from build123d import *

# Parameters (mm, degrees)
F1_DEPTH  = 26.8
F2_W      = 9.5
F2_H      = 26.8
F3_DEPTH  = 32.4
F4_W      = 53.02
F4_H      = 26.4
F5_DEPTH  = 15
F6_W      = 41.02
F6_H      = 26.4
F7_DEPTH  = 7
F8_W      = 33.1776287834
F8_H      = 14.4
F9_DEPTH  = 7
F10_W     = 16.1501816639
F10_H     = 14.4
F11_DEPTH = 7
F12_R     = 0.6930745825
F13_DEPTH = 5
F14_R     = 0.7453155857
F15_DEPTH = 5
F16_R     = 0.7584591481
F17_DEPTH = 5
F18_R     = 0.7431215043
F19_DEPTH = 5
F20_W     = 4
F20_H     = 9
F21_DEPTH = 5
F22_W     = 10
F22_H     = 13
F23_DEPTH = 1.5
F24_R     = 0.5
F25_R     = 2
F26_R     = 1
F27_DEPTH = 5
F28_R     = 1
F29_DEPTH = 5
F30_R     = 1
F31_DEPTH = 5
F32_R     = 1
F33_DEPTH = 5


with BuildPart() as f1:
    # F0 (on Front) → F1 (new body)
    with BuildSketch(Plane.XZ):
        Polygon((13.4, 0), (-13.4, 0), (-9.5, -6.25), (9.5, -6.25), align=None)
    extrude(amount=F1_DEPTH)

    # F2 (on face) → F3 (join)
    with BuildSketch(Plane(origin=(0, 0, -6.25), x_dir=(1, 0, 0), z_dir=(0, 0, -1))):
        Polygon((24, 42.91), (0, 42.91), (0, 26.8), (9.5, 26.8), (9.5, 0), (0, 0), (0, -16.11), (24, -16.11), align=None)
        with Locations((4.75, 13.4)):
            Rectangle(F2_W, F2_H)
    extrude(amount=F3_DEPTH)

    # F4 (on face) → F5 (cut)
    with BuildSketch(Plane.YZ.offset(24)):
        with Locations((-13.4, -22.45)):
            Rectangle(F4_W, F4_H)
    extrude(amount=-F5_DEPTH, mode=Mode.SUBTRACT)

    # F6 (on face) → F7 (cut)
    with BuildSketch(Plane.YZ.offset(9)):
        with Locations((-13.4, -22.45)):
            Rectangle(F6_W, F6_H)
    extrude(amount=-F7_DEPTH, mode=Mode.SUBTRACT)

    # F8 (on face) → F9 (cut)
    with BuildSketch(Plane.YZ.offset(9)):
        with Locations((-23.3211856083, -22.45)):
            Rectangle(F8_W, F8_H)
    extrude(amount=-F9_DEPTH, mode=Mode.SUBTRACT)

    # F10 (on face) → F11 (cut)
    with BuildSketch(Plane.YZ.offset(9)):
        with Locations((5.0349091681, -22.45)):
            Rectangle(F10_W, F10_H)
    extrude(amount=-F11_DEPTH, mode=Mode.SUBTRACT)

    # F12 (on face) → F13 (cut)
    with BuildSketch(Plane.YZ.offset(9)):
        with Locations((-36.91, -12.25)):
            Circle(F12_R)
    extrude(amount=-F13_DEPTH, mode=Mode.SUBTRACT)

    # F14 (on face) → F15 (cut)
    with BuildSketch(Plane.YZ.offset(9)):
        with Locations((10.11, -12.25)):
            Circle(F14_R)
    extrude(amount=-F15_DEPTH, mode=Mode.SUBTRACT)

    # F16 (on face) → F17 (cut)
    with BuildSketch(Plane.YZ.offset(9)):
        with Locations((-36.91, -32.65)):
            Circle(F16_R)
    extrude(amount=-F17_DEPTH, mode=Mode.SUBTRACT)

    # F18 (on face) → F19 (cut)
    with BuildSketch(Plane.YZ.offset(9)):
        with Locations((10.11, -32.65)):
            Circle(F18_R)
    extrude(amount=-F19_DEPTH, mode=Mode.SUBTRACT)

    # F20 (on face) → F21 (cut)
    with BuildSketch(Plane(origin=(0, 0, -38.65), x_dir=(1, 0, 0), z_dir=(0, 0, -1))):
        with Locations((11, 13.4)):
            Rectangle(F20_W, F20_H)
    extrude(amount=-F21_DEPTH, mode=Mode.SUBTRACT)

    # F22 (on face) → F23 (cut)
    with BuildSketch(Plane(origin=(0, 0, -38.65), x_dir=(1, 0, 0), z_dir=(0, 0, -1))):
        with Locations((10.75, 13.4)):
            Rectangle(F22_W, F22_H)
    extrude(amount=-F23_DEPTH, mode=Mode.SUBTRACT)

    # F24
    f24_edges = [f1.edges().sort_by_distance(p)[0] for p in [
        (5.75, -13.4, -38.65),
        (9, -13.4, -35.65),
        (13, -13.4, -37.15),
        (10.75, -6.9, -38.65),
        (11, -8.9, -37.15),
        (11, -17.9, -35.65),
        (15.75, -13.4, -38.65),
        (10.75, -19.9, -38.65),
    ]]
    fillet(f24_edges, radius=F24_R)

    # F25
    f25_edges = [f1.edges().sort_by_distance(p)[0] for p in [
        (0, -42.91, -22.45),
        (0, -13.4, -38.65),
        (0, 16.11, -22.45),
        (12, -42.91, -38.65),
        (12, -42.91, -6.25),
        (12, 16.11, -38.65),
        (12, 16.11, -6.25),
        (0, 8.055, -6.25),
        (0, -34.855, -6.25),
    ]]
    fillet(f25_edges, radius=F25_R)

    # F26 (on face) → F27 (cut)
    with BuildSketch(Plane(origin=(0, 0, -38.65), x_dir=(1, 0, 0), z_dir=(0, 0, -1))):
        with Locations((21.5, 37.41)):
            Circle(F26_R)
    extrude(amount=-F27_DEPTH, mode=Mode.SUBTRACT)

    # F28 (on face) → F29 (cut)
    with BuildSketch(Plane(origin=(0, 0, -38.65), x_dir=(1, 0, 0), z_dir=(0, 0, -1))):
        with Locations((21.5, -10.61)):
            Circle(F28_R)
    extrude(amount=-F29_DEPTH, mode=Mode.SUBTRACT)

    # F30 (on face) → F31 (cut)
    with BuildSketch(Plane.XY.offset(-6.25)):
        with Locations((21.5, 10.61)):
            Circle(F30_R)
    extrude(amount=-F31_DEPTH, mode=Mode.SUBTRACT)

    # F32 (on face) → F33 (cut)
    with BuildSketch(Plane.XY.offset(-6.25)):
        with Locations((21.5, -37.41)):
            Circle(F32_R)
    extrude(amount=-F33_DEPTH, mode=Mode.SUBTRACT)


solid = f1.part
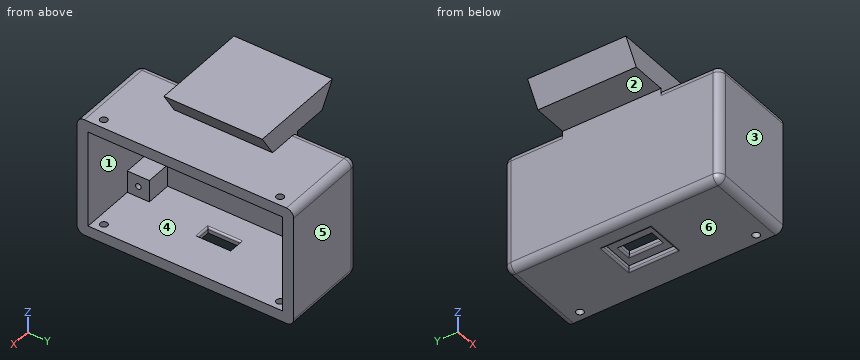
Could you check a few things on this model? Use its own coordinates, in mm. Face numbers are marked on the shaded views. A direction names the side the tool comes from. Coordinates: 2 decimals unless noted, no trailing zeros. Loops run counter-clockwise (first coordinate to the right, second up) from the corner with the lowest first, then second, coordinate; pieces in that order, holes last.
1. For P1, Ø0.8, axis at x = 11, z = -37.5, coming from the +Y side; P2, Ø1.7, axis at y = -37, z = -32.5, coming from the +X side; P3, Ø5, axis at x = 9, y = -12.5, coming from the -Z side; P4, Ø1.8, axis at x = 21.5, y = -37.41, coming from the +Z side, each with a flat end and sliding along its axis, tell me the tip position at first contact or that it passes through.
2. Imagine slicing it at B-B (x = 17.5). Please give me the cut outline in (y, z), and give its area (3 significant figures).
3. For the marked faces 1, 2 and 3, which set-ups out of +Z, -Z, +X, -X, +Y, -Y let a thin tool reach every point of the face, with its end or its side?
4. We'd pull the mould along Y, two halves only. Please class the marked faces 4, 5 and 6: released by +Y, released by -Y, zero draft, split by the parting line, or undercut.
5. Imagine slicing it at C-C (z = -10). Please give me the cut outline in (x, y).
6. Imagine slicing it at D-D (y = 5). Please give me the cut outline in (x, z), and give its area (3 significant figures).
7. I need wall thicknesses on L1, parallel to Y at x = 21.5, z = -36.5; L2, parallel to Z at x = 6.6, y = 10.11; L3, parallel to Y at x = 5.4, z = -32.65. Which ranges of each line are inside material? Lowest first, please.
8. Imagine slicing it at A-A (x = 21.5). Please give me the cut outline in (y, z), and give its area (3 significant figures).
Computed values:
1. P1: stops at y = 16.06
1. P2: stops at x = 9
1. P3: stops at z = -37.15
1. P4: passes through
2. outline: (-42.91, -36.65) arc R2 ccw to (-40.91, -38.65) - (14.11, -38.65) arc R2 ccw to (16.11, -36.65) - (16.11, -8.25) arc R2 ccw to (14.11, -6.25) - (-40.91, -6.25) arc R2 ccw to (-42.91, -8.25) - close; hole (-39.91, -35.65) - (13.11, -35.65) - (13.11, -9.25) - (-39.91, -9.25) - close
2. area: 509 mm2
3. face 1: +X
3. face 2: -Z, -X, +Y, -Y
3. face 3: +Z, -Z, +X, -X, -Y
4. face 4: undercut
4. face 5: released by +Y
4. face 6: zero draft
5. outline: (0, -40.91) arc R2 ccw to (2, -42.91) - (24, -42.91) - (24, -39.91) - (9, -39.91) - (9, -33.91) - (2, -33.91) - (2, 7.11) - (9, 7.11) - (9, 13.11) - (24, 13.11) - (24, 16.11) - (2, 16.11) arc R2 ccw to (0, 14.11) - close
6. outline: (0, -36.65) arc R2 ccw to (2, -38.65) - (24, -38.65) - (24, -35.65) - (2, -35.65) - (2, -9.25) - (24, -9.25) - (24, -6.25) - (2, -6.25) arc R2 ccw to (0, -8.25) - close
6. area: 195 mm2
7. L1: y = -42.91 to -38.41, -36.41 to 9.61, 11.61 to 16.11
7. L2: z = -38.65 to -33.39, -31.91 to -29.65, -15.25 to -13, -11.5 to -6.25
7. L3: y = -42.91 to -37.67, -36.15 to -33.91, 7.11 to 9.37, 10.85 to 16.11
8. outline: (-42.91, -36.65) arc R2 ccw to (-40.91, -38.65) - (-38.41, -38.65) - (-38.41, -35.65) - (-39.91, -35.65) - (-39.91, -9.25) - (-38.41, -9.25) - (-38.41, -6.25) - (-40.91, -6.25) arc R2 ccw to (-42.91, -8.25) - close; (-36.41, -38.65) - (9.61, -38.65) - (9.61, -35.65) - (-36.41, -35.65) - close; (-36.41, -9.25) - (9.61, -9.25) - (9.61, -6.25) - (-36.41, -6.25) - close; (11.61, -38.65) - (14.11, -38.65) arc R2 ccw to (16.11, -36.65) - (16.11, -8.25) arc R2 ccw to (14.11, -6.25) - (11.61, -6.25) - (11.61, -9.25) - (13.11, -9.25) - (13.11, -35.65) - (11.61, -35.65) - close
8. area: 485 mm2
